Input: part model. Units: mm. Frame: model coordinates. Face numbers are marked on the shaded views. A direction names the side the tool comes from. Coordinates: 2 decimals unless noted, no trailing zeros. Write each loop counter-clockwise with the first axis right and the second up, starting at its lowest first coordinate (ties: lowest second). Pieces come first, ordered by that corner, then holes. Notation, with made-up numbers: M 87,62 L 109,62 A16 ccw 109,82 Z; hole C 87.5,24.5 d10. An arc over 180 degrees is marked long. Write each question's results on one line, items separated by ' | '. Start each with the question number.
1. Section query B-B, the plane z = 0. Output: boundary loops of the cut face in (x, y).
2. Set-up query: the marked faces 1, 2 and 3. Return all of +Z, -Z, +X, -X, +Y, -Y with unobstructed straight access to the full face (end or side cutting, diameter ignored); none if empty.
3. Section query A-A, the plane y = 15.5. Output: boundary loops of the cut face in (x, z).
4. Section query C-C, the plane y = 11. Output: boundary loops of the cut face in (x, z).
5. Ray query, probe 1 along Z at (x, y) = (3.5, 4); probe 2 along Z at (x, y) = (-15.5, 6.5); probe 3 along Y at (x, z) = (-19.5, 2.75). Return the intervals inside material, ascending.
6. First-contact query: pin 1 (1.5 mm diameter, centred on y = 6, z = 2.5, fed in from -X); pin 2 (3 mm diameter, centred on y = 19, z = 0.5, fed in from +X); pin 3 (0.8 mm diameter, centred on x = -10, z = -1.5, fed in from +Y). Flat tips, straight axial feed; report the tip coordinate or a pass-through.
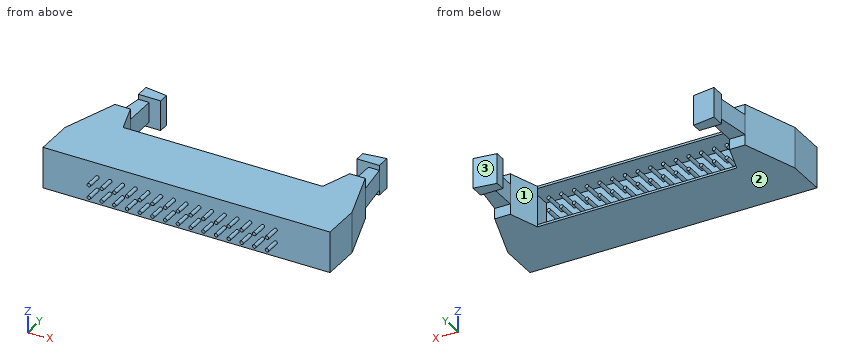
```python
from build123d import *

# Parameters (mm, degrees)
EXTRUDE_1_DEPTH      = 4.1
EXTRUDE_1_DEPTH_BACK = 4.1
SKETCH_3_W           = 42
SKETCH_3_H           = 7.294129616
CUT_EXTRUDE_1_DEPTH  = 5
EXTRUDE_2_DEPTH      = 2
EXTRUDE_2_DEPTH_BACK = 2
EXTRUDE_3_DEPTH      = 3
EXTRUDE_3_DEPTH_BACK = 3
EXTRUDE_4_DEPTH      = 3
EXTRUDE_4_DEPTH_BACK = 12.5
SKETCH_6_R           = 0.35


with BuildPart() as part:
    # Эскиз2 → Бобышка-Вытянуть1 (new, two sides: drawn at the far end of the back side and taken through both)
    with BuildSketch(Plane.XY.offset(-EXTRUDE_1_DEPTH_BACK)):
        Polygon((21.889579694, 14.852543655), (19.907114806, 8.85), (-19.907114806, 8.85), (-21.889579694, 14.852543655), (-24.992568214, 14.852543655), (-28.65, 3.85), (-28.65, -3.85), (28.65, -3.85), (28.65, 3.85), (24.992568214, 14.852543655), align=None)
    extrude(amount=EXTRUDE_1_DEPTH + EXTRUDE_1_DEPTH_BACK)

    # Эскиз3 → Вырез-Вытянуть1 (cut)
    with BuildSketch(Plane(origin=(0, 8.85, 0), x_dir=(1, 0, 0), z_dir=(0, 1, 0))):
        Rectangle(SKETCH_3_W, SKETCH_3_H)
    extrude(amount=-CUT_EXTRUDE_1_DEPTH, mode=Mode.SUBTRACT)

    # Эскиз4 → Бобышка-Вытянуть2 (add, two sides: drawn at the far end of the back side and taken through both)
    with BuildSketch(Plane.XY.offset(-EXTRUDE_2_DEPTH_BACK)):
        Polygon((-24.992568214, 14.852543655), (-21.889579694, 14.852543655), (-21.889579694, 21.400452047), (-24.052396461, 21.400452047), align=None)
        Polygon((24.052396461, 21.400452047), (24.992568214, 14.852543655), (21.889579694, 14.852543655), (21.889579694, 21.400452047), align=None)
    extrude(amount=EXTRUDE_2_DEPTH + EXTRUDE_2_DEPTH_BACK)

    # Эскиз5 → Бобышка-Вытянуть3 (add, two sides: drawn at the far end of the back side and taken through both)
    with BuildSketch(Plane.XY.offset(-EXTRUDE_3_DEPTH_BACK)):
        Polygon((-24.052396461, 21.400452047), (-24.052396461, 24.074868015), (-19.60201978, 23.435867253), (-19.60201978, 21.400452047), (-21.889579694, 21.400452047), align=None)
        Polygon((19.60201978, 21.400452047), (21.889579694, 21.400452047), (24.052396461, 21.400452047), (24.052396461, 24.074868015), (19.60201978, 23.435867253), align=None)
    extrude(amount=EXTRUDE_3_DEPTH + EXTRUDE_3_DEPTH_BACK)

    # Эскиз6 → Бобышка-Вытянуть4 (add, two sides: drawn at the far end of the back side and taken through both)
    with BuildSketch(Plane.XZ.offset(3.85).offset(-EXTRUDE_4_DEPTH_BACK)):
        with Locations((0, 1.27)):
            Circle(SKETCH_6_R)
        with Locations((0, -1.27)):
            Circle(SKETCH_6_R)
        with Locations((2.54, -1.27)):
            Circle(SKETCH_6_R)
        with Locations((2.54, 1.27)):
            Circle(SKETCH_6_R)
        with Locations((5.08, -1.27)):
            Circle(SKETCH_6_R)
        with Locations((5.08, 1.27)):
            Circle(SKETCH_6_R)
        with Locations((7.62, -1.27)):
            Circle(SKETCH_6_R)
        with Locations((7.62, 1.27)):
            Circle(SKETCH_6_R)
        with Locations((10.16, -1.27)):
            Circle(SKETCH_6_R)
        with Locations((10.16, 1.27)):
            Circle(SKETCH_6_R)
        with Locations((12.7, -1.27)):
            Circle(SKETCH_6_R)
        with Locations((12.7, 1.27)):
            Circle(SKETCH_6_R)
        with Locations((15.24, -1.27)):
            Circle(SKETCH_6_R)
        with Locations((15.24, 1.27)):
            Circle(SKETCH_6_R)
        with Locations((17.78, -1.27)):
            Circle(SKETCH_6_R)
        with Locations((17.78, 1.27)):
            Circle(SKETCH_6_R)
        with Locations((-2.54, -1.27)):
            Circle(SKETCH_6_R)
        with Locations((-2.54, 1.27)):
            Circle(SKETCH_6_R)
        with Locations((-5.08, -1.27)):
            Circle(SKETCH_6_R)
        with Locations((-5.08, 1.27)):
            Circle(SKETCH_6_R)
        with Locations((-7.62, -1.27)):
            Circle(SKETCH_6_R)
        with Locations((-7.62, 1.27)):
            Circle(SKETCH_6_R)
        with Locations((-10.16, -1.27)):
            Circle(SKETCH_6_R)
        with Locations((-10.16, 1.27)):
            Circle(SKETCH_6_R)
        with Locations((-12.7, -1.27)):
            Circle(SKETCH_6_R)
        with Locations((-12.7, 1.27)):
            Circle(SKETCH_6_R)
        with Locations((-15.24, -1.27)):
            Circle(SKETCH_6_R)
        with Locations((-15.24, 1.27)):
            Circle(SKETCH_6_R)
        with Locations((-17.78, -1.27)):
            Circle(SKETCH_6_R)
        with Locations((-17.78, 1.27)):
            Circle(SKETCH_6_R)
    extrude(amount=EXTRUDE_4_DEPTH + EXTRUDE_4_DEPTH_BACK)


solid = part.part
```
Answer:
1) outline: M -28.65,-3.85 L 28.65,-3.85 L 28.65,3.85 L 24.99,14.85 L 24.05,21.4 L 24.05,24.07 L 19.6,23.44 L 19.6,21.4 L 21.89,21.4 L 21.89,14.85 L 19.91,8.85 L 21,8.85 L 21,3.85 L -21,3.85 L -21,8.85 L -19.91,8.85 L -21.89,14.85 L -21.89,21.4 L -19.6,21.4 L -19.6,23.44 L -24.05,24.07 L -24.05,21.4 L -24.99,14.85 L -28.65,3.85 Z
2) face 1: +Z, -Z | face 2: -Z, +X, -X, +Y, -Y | face 3: +Z, -Z, +Y
3) outline: M -24.9,-2 L -21.89,-2 L -21.89,2 L -24.9,2 Z; M 21.89,-2 L 24.9,-2 L 24.9,2 L 21.89,2 Z
4) outline: M -26.27,-4.1 L -20.62,-4.1 L -20.62,4.1 L -26.27,4.1 Z; M 20.62,-4.1 L 26.27,-4.1 L 26.27,4.1 L 20.62,4.1 Z
5) probe 1: -4.1 to -3.65, 3.65 to 4.1 | probe 2: -4.1 to -3.65, -1.5 to -1.04, 1.04 to 1.5, 3.65 to 4.1 | probe 3: -3.85 to 3.85
6) pin 1: x = -28.18 | pin 2: x = 24.61 | pin 3: y = 8.65
